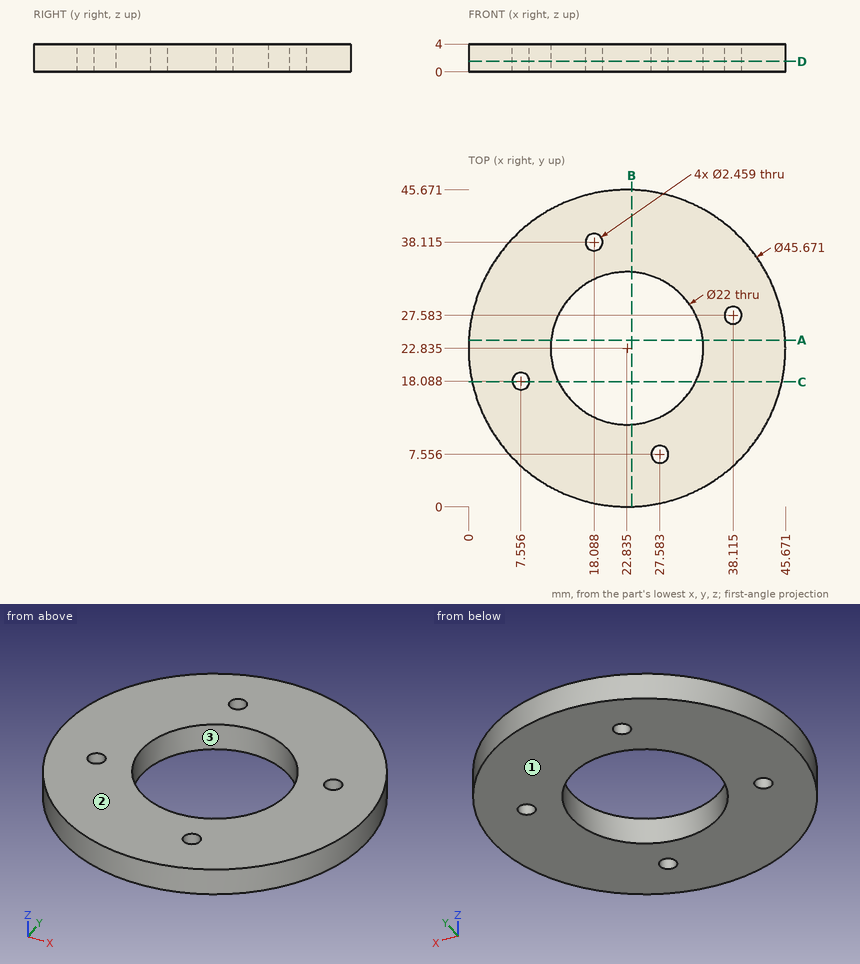
Drawing for the job (mm, zero at the part's lowest x, y, z). Round coordinates to 2 decimals unless told otherwise and drop trailing zeros. Write each loop counter-clockwise with the first axis right and the second up, starting at its lowest first coordinate (ties: lowest second). Pieces come first, ordered by that corner, then holes. Notation, with made-up numbers: (4.25, -32.5) - (61.25, -32.5) arc R29 cw to (61.25, -2.5) - close; hole circle Ø6 at (8, -3). An arc over 180 degrees is marked (long way). Use CSV: the item, a comma, the result in double quotes.
(1) Band-saw the part on A-A (y = 24). Write the cut outline in (x, z).
Response:
outline,"(0.03, 0) - (11.9, 0) - (11.9, 4) - (0.03, 4) - close; (33.77, 0) - (45.64, 0) - (45.64, 4) - (33.77, 4) - close"
(2) Band-saw the part on C-C (y = 18). Write the cut outline in (x, z) (1 decimal).
Response:
outline,"(0.5, 0) - (6.3, 0) - (6.3, 4) - (0.5, 4) - close; (8.8, 0) - (13, 0) - (13, 4) - (8.8, 4) - close; (32.7, 0) - (45.2, 0) - (45.2, 4) - (32.7, 4) - close"
(3) Band-saw the part on B-B (x = 23.5). Write the cut outline in (y, z) (1 decimal).
Response:
outline,"(0, 0) - (11.9, 0) - (11.9, 4) - (0, 4) - close; (33.8, 0) - (45.7, 0) - (45.7, 4) - (33.8, 4) - close"
(4) Pin check, flat tips, straight feed: P1, Ø1.5, axis at x = 18, z = 3.5, coming from the -Y side; P2, Ø1, axis at y = 16, z = 2, coming from the -X side; P3, Ø2, axis at x = 38.11, y = 27.58, coming from the +Z side; P4, Ø4, axis at x = 7.56, y = 18.09, coming from the -Z side. Stop position of each tip, or through.
Response:
P1,"y = 0.37"
P2,"x = 0.9"
P3,"through"
P4,"z = 0"
(5) Wall check: line 1 (X direction, y = 28.5, z = 3.5) (1 decimal); line 2 (Y direction, x = 27, z = 0.2) (1 decimal); line 3 (X direction, y = 27.5, z = 0.8) (1 decimal). Give the ranges that are in metal, low to high.
Response:
line 1,"0.7 to 13.4, 32.3 to 37.3, 38.9 to 45"
line 2,"0.4 to 6.5, 8.6 to 12.7, 33 to 45.3"
line 3,"0.5 to 12.9, 32.8 to 36.9, 39.3 to 45.2"
(6) Mould opens along Z. For the marked faces 1, 2 and 3 say: pulls with the +Z half, pulls with the -Z half, needs draft (parallel to the pull), parting line crosses it, or undercut.
Response:
face 1,"pulls with the -Z half"
face 2,"pulls with the +Z half"
face 3,"needs draft"
(7) Band-saw the part on D-D (z = 1.5). Write the cut outline in (x, y) (1 decimal).
Response:
outline,"circle Ø45.7 at (22.8, 22.8); hole circle Ø2.5 at (7.6, 18.1); hole circle Ø22 at (22.8, 22.8); hole circle Ø2.5 at (18.1, 38.1); hole circle Ø2.5 at (27.6, 7.6); hole circle Ø2.5 at (38.1, 27.6)"
